Work out the finished part from the listing and answer in its coordinate system (mm). Face numbers are marked on the shaded views. A direction names the side the tool comes from. Round coordinates to 2 decimals unless told otherwise and drop trailing zeros. Order: outer loops, then holes, each group sorted by start corner. A loop starts at its lowest first (then second) coordinate and runs counter-clockwise, first axis right, second up. Notation, with made-up numbers: (63.25, -21.5) - (121.25, -21.5) arc R18 cw to (121.25, 12.5) - close; hole circle Ø10 at (-28.75, 55.5). An arc over 180 degrees is marked (long way). Use one line per item in the form item = value. Start each with the question number.
Q1. The part is cut by section A-A on y = 14.5. Determine the outline of the cut face in (x, z) (3 decimals).
Q2. Which of the six approach directions +Z, -Z, +X, -X, +Y, -Y give full straight-line access (tool end or side, diameter ignored) to the marked faces 4, 5, 6 and 7?
Q3. Find the intervals of material crossed by line 1 (X direction, y = 4.5, z = -0.25) (3 decimals); line 2 (X direction, y = 11.75, z = -1) (3 decimals); line 3 (Z direction, x = -6, y = 2.5), in increasing order. Write a range as [from, to].
Q4. The part is cut by section D-D on y = 4. Determine the outline of the cut face in (x, z) (3 decimals), plus the area to 3 significant figures.
Q5. Given P1, Ø2, axis at x = -10, y = 4, coming from the -Z side; P2, Ø0.6, axis at y = -1, z = -1, coming from the -X side; P3, Ø2, axis at x = -7.5, z = -3, coming from the -Y side; P4, Ø8, axis at y = 0, z = 1, coming from the -X side (3 decimals), each flat-ended and moving along its own axis, determine where each tip first touches the part or whether it passes through.
Q6. For a pull along X with two mould halves and no side action, classify the marked faces 1, 2 and 3 as +X half, -X half, draft (parallel to the pull), parting line (faces both ways), or undercut.
Q7. The part is cut by section B-B on z = -5. Determine the outline of the cut face in (x, y) (3 decimals), plus the area to 3 significant figures.
Q8. The part is cut by section C-C on x = 8. Determine the outline of the cut face in (y, z).
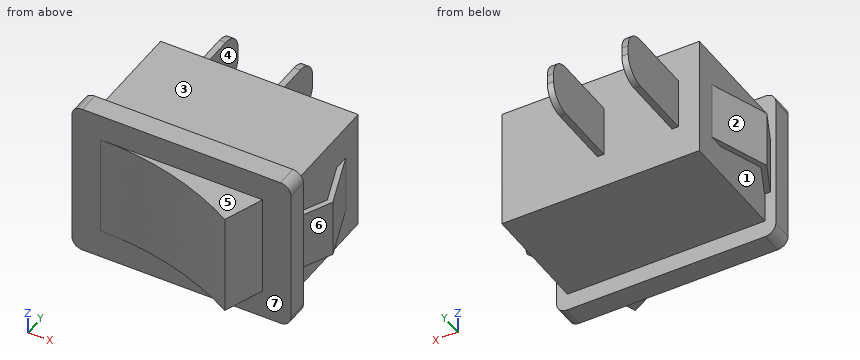
from build123d import *

# Parameters (mm, degrees)
SKETCH1_W           = 18.75
SKETCH1_H           = 11.52
BOSS_EXTRUDE1_DEPTH = 10.6
SKETCH2_W           = 20.8
SKETCH2_H           = 14.82
BOSS_EXTRUDE2_DEPTH = 2
BOSS_EXTRUDE3_START = -2.5
BOSS_EXTRUDE3_DEPTH = 9.6
SKETCH5_W           = 0.6
SKETCH5_H           = 4.85
BOSS_EXTRUDE4_DEPTH = 8.1
BOSS_EXTRUDE5_START = -2.85
BOSS_EXTRUDE5_DEPTH = 5.5
FILLET1_R           = 2
FILLET2_R           = 1


with BuildPart() as part:
    # Sketch1 → Boss-Extrude1 (new body)
    with BuildSketch(Plane(origin=(0, 0, 0), x_dir=(1, 0, 0), z_dir=(0, 1, 0))):
        Rectangle(SKETCH1_W, SKETCH1_H)
    extrude(amount=BOSS_EXTRUDE1_DEPTH)

    # Sketch2 → Boss-Extrude2 (add)
    with BuildSketch(Plane(origin=(0, 0, 0), x_dir=(1, 0, 0), z_dir=(0, 1, 0))):
        Rectangle(SKETCH2_W, SKETCH2_H)
    extrude(amount=-BOSS_EXTRUDE2_DEPTH)

    # Sketch4 → Boss-Extrude3 (add)
    with BuildSketch(Plane.XY.offset(7.41).offset(BOSS_EXTRUDE3_START)):
        with BuildLine():
            Line((7.7, -2), (-7.7, -2))
            add(Edge.make_bspline(
                [(-7.7, -2), (-0.364289246, -2.017203107), (6.331919427, -5.758770483)],
                knots=[0, 0, 0, 1, 1, 1], degree=2))
            Line((6.331919427, -5.758770483), (7.7, -2))
        make_face()
    extrude(amount=-BOSS_EXTRUDE3_DEPTH)

    # Sketch5 → Boss-Extrude4 (add)
    with BuildSketch(Plane(origin=(0, 10.6, 0), x_dir=(1, 0, 0), z_dir=(0, 1, 0))):
        with Locations((-7.075, 0)):
            Rectangle(SKETCH5_W, SKETCH5_H)
        Rectangle(SKETCH5_W, SKETCH5_H)
    extrude(amount=BOSS_EXTRUDE4_DEPTH)

    # Sketch6 → Boss-Extrude5 (add)
    with BuildSketch(Plane(origin=(0, 0, -5.76), x_dir=(-1, 0, 0), z_dir=(0, 0, -1)).offset(BOSS_EXTRUDE5_START)):
        Polygon((11.375, 3.105045161), (9.375, 8.6), (9.375, 7.1380978), (10.833272639, 3.131526652), (9.436573077, 0.216020625), (9.375, 0.087491424), (9.375, 0), (9.8875, 0), align=None)
    boss_extrude5 = extrude(amount=-BOSS_EXTRUDE5_DEPTH)

    # Mirror1: Boss-Extrude5 across plane
    add(boss_extrude5.mirror(Plane(origin=(0, 0, 0), x_dir=(0, 0, 1), z_dir=(1, 0, 0))))

    # Fillet1
    fillet1_edges = [part.edges().sort_by_distance(p)[0] for p in [
        (-7.075, 18.7, -2.425),
        (-7.075, 18.7, 2.425),
        (0, 18.7, -2.425),
        (0, 18.7, 2.425),
    ]]
    fillet(fillet1_edges, radius=FILLET1_R)

    # Fillet2
    fillet2_edges = [part.edges().sort_by_distance(p)[0] for p in [
        (10.4, -1, -7.41),
        (10.4, -1, 7.41),
        (-10.4, -1, 7.41),
        (-10.4, -1, -7.41),
    ]]
    fillet(fillet2_edges, radius=FILLET2_R)


solid = part.part
Found:
q1.outline = (-7.375, -2.425) - (-6.775, -2.425) - (-6.775, 2.425) - (-7.375, 2.425) - close; (-0.3, -2.425) - (0.3, -2.425) - (0.3, 2.425) - (-0.3, 2.425) - close
q2.face_4 = +Z, -Z, +Y
q2.face_5 = +Z, +X, -X, -Y
q2.face_6 = +Z, -Z, +X
q2.face_7 = -Y
q3.line_1 = [-10.867, -10.335], [-9.375, 9.375], [10.335, 10.867]
q3.line_2 = [-7.375, -6.775], [-0.3, 0.3]
q3.line_3 = [-5.76, 5.76]
q4.outline = (-11.049, -2.91) - (-10.517, -2.91) - (-10.517, 2.59) - (-11.049, 2.59) - close; (-9.375, -5.76) - (9.375, -5.76) - (9.375, 5.76) - (-9.375, 5.76) - close; (10.517, -2.91) - (11.049, -2.91) - (11.049, 2.59) - (10.517, 2.59) - close
q4.area = 222 mm²
q5.P1 = -5.76
q5.P2 = -10.4
q5.P3 = -2.03
q5.P4 = -11.375
q6.face_1 = undercut
q6.face_2 = -X half
q6.face_3 = draft
q7.outline = (-10.4, -2) - (10.4, -2) - (10.4, 0) - (9.375, 0) - (9.375, 10.6) - (-9.375, 10.6) - (-9.375, 0) - (-10.4, 0) - close
q7.area = 240 mm²
q8.outline = (-2, -7.41) - (0, -7.41) - (0, -5.76) - (10.6, -5.76) - (10.6, 5.76) - (0, 5.76) - (0, 7.41) - (-2, 7.41) - close
